Autodesk Inventor part; units mm, degrees
ref_plane "YZ Plane" through (0, 0, 0) normal (1, 0, 0) x (0, 1, 0)
ref_plane "XZ Plane" through (0, 0, 0) normal (0, 1, 0) x (-1, 0, 0)
ref_plane "XY Plane" through (0, 0, 0) normal (0, 0, 1) x (1, 0, 0)
sketch "Esboço1" plane through (0, 0, 0) normal (0, 1, 0) x (-1, 0, 0)
  circle A0 centre (0, 0) radius 5
  dimension "d0" = 10
extrude "Extrusão1" add sketch "Esboço1" along normal blind 80
sketch "Esboço3" plane through (0, 0, 0) normal (0, -1, 0) x (1, 0, 0)
  circle A0 centre (0, 0) radius 2.5
  dimension "d9" = 5
extrude "Extrusão3" add sketch "Esboço3" along normal blind 6
thread "Rosca2"
sketch "Sketch4" plane through (0, 80, 0) normal (0, 1, 0) x (1, 0, 0)
  circle A0 centre (0, 0) radius 5
hole "Hole1" at (0, 80, 0) direction (0, -1, 0) diameter 4.134 depth 14.2 tip angle 118
equation "\"Raio_vergadura\" = Espessura"
equation "\"Largura_alívio_de_vergadura\" = Espessura"
equation "\"Profundidade_alívio_de_vergadura\" = 0.5 * Espessura"
equation "\"Tamanho_alívio_de_dobra\" = 4 * Espessura"
equation "\"Remanescente_mínimo\" = 2 * Espessura"
equation "\"Raiodetransição\" = Raio_vergadura"
equation "\"Tamanho_de_raio_de_Jacobi\" = Raio_vergadura"
equation "\"TamanhoFolga\" = Espessura"
properties part number "Suporte da mesa" material "Brass, Soft Yellow"
Check sheet for the modelled part. Datum: model origin and axes. Units: mm. A direction names the side the tool comes from. Round coordinates to 2 decimals unless told otherwise and drop trailing zeros. Write each loop counter-clockwise with the first axis right and the second up, starting at its lowest first coordinate (ties: lowest second). Pieces come first, ordered by that corner, then holes. Notation, with made-up numbers: (63.5, 46.25) -> (111.5, 46.25) arc R22 cw to (111.5, 61.25) -> close; hole circle Ø2 at (70.5, 81.5). An arc over 180 degrees is marked (long way). One line per question, with ' | ' between items. Start each with the question number.
1. Set-up check for faces 1 (the face through (-2, 0, -2)), 2 (the face through (1.26, 72.8, -1.64)), 3 (the face through (0, -6, 0)): record each of +Z, -Z, +X, -X, +Y, -Y from which the full face is reachable in a straight line by a thin tool's end or side.
2. Sectioned sample at A-A, the plane y = 67.5. Record the cut outline in (x, z), then the cut area to 3 significant figures.
3. Sectioned sample at D-D, the plane z = 3.5. Record the cut outline in (x, y), then the cut area to 3 significant figures.
4. Depth check by flat-ended pin: pin 1 (5 mm diameter, centred on x = -3, y = 60, fed in from +Z); pin 2 (1.5 mm diameter, centred on y = 19.5, z = 3, fed in from -X); pin 3 (6 mm diameter, centred on y = 44, z = 3.5, fed in from +X). Enter the tip coordinate at first touch or a pass-through.
5. Scan lines: line 1 along Z through (x, y) = (0, 73.5); line 2 along Y through (x, z) = (2, -3.75); line 3 along Z through (x, y) = (3.75, 18.5). Record each from-to range of solid material in increasing order. Write a range as from..to.
6. Release check for a two-part mould opening along Z. For faces 4 (the face through (-0.137, 64.774, 0.332)), 5 (the face through (-2, 80, -1)), 6 (the face through (-0.54, -2.96, 2.44)) record: +Z half, -Z half, draft (parallel to the pull), parting line (faces both ways), or undercut.
7. Sectioned sample at B-B, the plane y = 3. Record the cut outline in (x, z), then the cut area to 3 significant figures.
8. Sectioned sample at C-C, the plane x = 3.25. Record the cut outline in (y, z).
Taken from the geometry:
1) face 1: -Y | face 2: +Y | face 3: +Z, -Z, +X, -X, -Y
2) outline: circle Ø10 at (0, 0); hole circle Ø4.13 at (0, 0) | area: 65.1 mm^2
3) outline: (-3.57, 0) -> (3.57, 0) -> (3.57, 80) -> (-3.57, 80) -> close | area: 571 mm^2
4) pin 1: stops at z = 4.97 | pin 2: stops at x = -4.47 | pin 3: stops at x = 4.97
5) line 1: z = -5..-2.07, 2.07..5 | line 2: y = 0..80 | line 3: z = -3.31..3.31
6) face 4: undercut | face 5: draft | face 6: parting line
7) outline: circle Ø10 at (0, 0) | area: 78.5 mm^2
8) outline: (0, -3.8) -> (80, -3.8) -> (80, 3.8) -> (0, 3.8) -> close
